from build123d import *

# Parameters (mm, degrees)
BOX_W        = 141
BOX_H        = 73.6
BOX_DEPTH    = 22.5
FILLET_R     = 3
BOX004_W     = 5
BOX004_H     = 75.6
BOX004_DEPTH = 23.5
FILLET004_R  = 4


with BuildPart() as battery_fillet:
    # Box → Box (new body)
    with BuildSketch(Plane(origin=(2, 0, 0), x_dir=(1, 0, 0), z_dir=(0, 0, 1))):
        with Locations((70.5, 36.8)):
            Rectangle(BOX_W, BOX_H)
    extrude(amount=BOX_DEPTH)

    # Fillet
    fillet_edges = [battery_fillet.edges().sort_by_distance(p)[0] for p in [
        (72.5, 0, 0),
        (72.5, 0, 22.5),
        (72.5, 73.6, 0),
        (72.5, 73.6, 22.5),
    ]]
    fillet(fillet_edges, radius=FILLET_R)


with BuildPart() as battery_fillet_1:
    # Fillet placement: moved
    add(battery_fillet.part.moved(Location((0, -36.8, 0))))


with BuildPart() as test_back_wall_cut:
    # Box004 → Box004 (new body)
    with BuildSketch(Plane(origin=(1.5, -37.8, 0), x_dir=(1, 0, 0), z_dir=(0, 0, 1))):
        with Locations((2.5, 37.8)):
            Rectangle(BOX004_W, BOX004_H)
    extrude(amount=BOX004_DEPTH)

    # Fillet004
    fillet004_edges = [test_back_wall_cut.edges().sort_by_distance(p)[0] for p in [
        (4, -37.8, 23.5),
        (4, 37.8, 23.5),
    ]]
    fillet(fillet004_edges, radius=FILLET004_R)

    # Cut003: cut battery fillet
    add(battery_fillet_1.part, mode=Mode.SUBTRACT)


solid = test_back_wall_cut.part
Work out the finished part from the listing and answer in its coordinate system (mm). A direction names the side the tool comes from. Give positions to 0.01 mm unless a question says otherwise; leave off trailing zeros. Write each loop counter-clockwise with the first axis right and the second up, starting at its lowest first coordinate (ties: lowest second). Pieces come first, ordered by that corner, then holes.
Q1. The part is cut by section A-A on x = 5.35. Give the vertices of the cut face in (y, z), and give its area (3 significant figures).
Answer:
outline: (-37.8, 0) - (-33.8, 0) arc R3 cw to (-36.8, 3) - (-36.8, 19.5) arc R3 cw to (-33.8, 22.5) - (33.8, 22.5) arc R3 cw to (36.8, 19.5) - (36.8, 3) arc R3 cw to (33.8, 0) - (37.8, 0) - (37.8, 19.5) arc R4 ccw to (33.8, 23.5) - (-33.8, 23.5) arc R4 ccw to (-37.8, 19.5) - close
area: 121 mm2
Q2. The part is cut by section C-C on y = -12.5. Give the vertices of the cut face in (x, z), and give its area (4 significant figures).
Answer:
outline: (1.5, 0) - (2, 0) - (2, 22.5) - (6.5, 22.5) - (6.5, 23.5) - (1.5, 23.5) - close
area: 16.25 mm2
Q3. A tool of negligible diameter and unlimited length cuts with its end or side. For faces 1 (the face through (4.28, 35.94, 0.9)), 2 (the face through (4, -37.8, 10)), from which of +Z, -Z, +X, -X, +Y, -Y can it reach the whole face along a straight path? Write none if from no direction.
Answer:
face 1: +X
face 2: +Z, -Z, +X, -X, -Y
Q4. Given pin 1 (2 mm diameter, centred on x = 4, y = 5.5, fed in from -Z); pin 2 (11 mm diameter, centred on y = -0.5, z = 11.5, fed in from +X), each flat-ended and moving along its own axis, determine where each tip first touches the part or whether it passes through.
Answer:
pin 1: stops at z = 22.5
pin 2: stops at x = 2
Q5. For a pull along Z with two mould halves and no side action, classify faces 3 (the face through (4, 0, 22.5)), 4 (the face through (4.035, 36.659, 22.297)), 5 (the face through (4.28, -35.94, 21.6)) as released by +Z, released by -Z, zero draft, split by the parting line, or undercut.
Answer:
face 3: released by -Z
face 4: released by +Z
face 5: undercut
Q6. The part is cut by section B-B on z = 4.5. Give the vertices of the cut face in (x, y), and give its area (3 significant figures).
Answer:
outline: (1.5, -37.8) - (6.5, -37.8) - (6.5, -36.8) - (2, -36.8) - (2, 36.8) - (6.5, 36.8) - (6.5, 37.8) - (1.5, 37.8) - close
area: 46.8 mm2
Q7. Straight lines are drawn through the part: L1, parallel to Y at x = 2.05, z = 6; L2, parallel to X at y = -3, z = 4.5; L3, parallel to Z at x = 2.2, y = 17. For each, find the intervals that lie inside material, in ascending order.
Answer:
L1: y = -37.8 to -36.8, 36.8 to 37.8
L2: x = 1.5 to 2
L3: z = 22.5 to 23.5
